Build history of the part. All positions in model axes, mm. Give positions to 0.01 mm unless a question says otherwise; leave off trailing zeros. Order: outer loops, then holes, each group sorted by start corner. A loop starts at its lowest first (then second) coordinate and runs counter-clockwise, first axis right, second up. Notation, with made-up numbers: M -26,52.25 L 5,52.25 A20 cw 5,58.25 Z; hole C 26.25,-8 d8. An arc over 180 degrees is marked long. One line per item, written item: value. Start each with the question number.
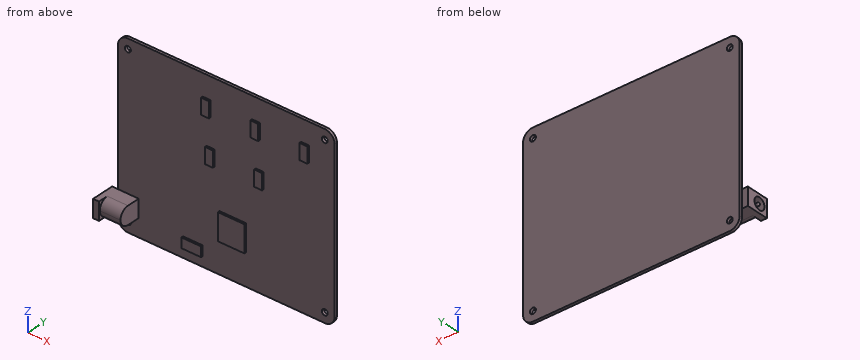
Autodesk Inventor part; units mm, degrees
ref_plane "YZ Plane" through (0, 0, 0) normal (1, 0, 0) x (0, 1, 0)
ref_plane "XZ Plane" through (0, 0, 0) normal (0, 1, 0) x (-1, 0, 0)
ref_plane "XY Plane" through (0, 0, 0) normal (0, 0, 1) x (1, 0, 0)
sketch "草圖1" plane through (0, 0, 0) normal (0, 1, 0) x (-1, 0, 0)
  line L0 (0, 0) -> (110, 0)
  line L1 (110, 0) -> (110, 90)
  line L2 (110, 90) -> (0, 90)
  line L3 (0, 90) -> (0, 0)
  dimension "d0" = 110
  dimension "d1" = 90
extrude "擠出1" add sketch "草圖1" along normal blind 1.4
fillet "圓角1" radius 5 4 edges at (0, 0.7, 90) (0, 0.7, 0) (-110, 0.7, 90) (-110, 0.7, 0)
sketch "草圖2" plane through (0, 0, 0) normal (0, -1, 0) x (1, 0, 0)
  line L0 (-5, 0) -> (-105, 0)
  line L1 (0, 85) -> (0, 5)
  line L2 (-105, 90) -> (-5, 90)
  line L3 (-110, 5) -> (-110, 85)
  point P0 (0, 0)
  point P1 (-105, 85)
  point P2 (-105, 5)
  point P3 (-5, 85)
  point P4 (-5, 5)
  dimension "d5" = 5
  dimension "d6" = 5
  dimension "d7" = 5
  dimension "d8" = 5
hole "孔1" at (-105, 0, 85) at (-105, 0, 5) at (-5, 0, 85) at (-5, 0, 5) direction (0, 1, 0) diameter 3 end through all
sketch "草圖3" plane through (0, 0, 0) normal (0, -1, 0) x (1, 0, 0)
  line L0 (-5, 0) -> (-105, 0)
  line L1 (-110, 5) -> (-110, 85)
  line L2 (-113, 18) -> (-99.5, 18)
  line L3 (-99.5, 18) -> (-99.5, 9)
  line L4 (-99.5, 9) -> (-113, 9)
  line L5 (-113, 9) -> (-113, 18)
  point P0 (0, 0)
  dimension "d16" = 9
  dimension "d17" = 9
  dimension "d18" = 13.5
  dimension "d19" = 3
extrude "擠出2" add sketch "草圖3" along normal blind 11
sketch "草圖5" plane through (0, -11, 0) normal (0, -1, 0) x (1, 0, 0)
  line L0 (-113, 9) -> (-99.5, 9)
  line L1 (-113, 18) -> (-110, 18)
  line L2 (-110, 18) -> (-110, 9)
  line L3 (-110, 9) -> (-113, 9)
  line L4 (-113, 9) -> (-113, 18)
  point P0 (0, 0)
  dimension "d23" = 3
extrude "擠出3" add sketch "草圖5" along normal blind 0.5
fillet "圓角2" radius 4.5 2 edges at (-104.75, -11, 18) (-104.75, -11, 9)
sketch "草圖7" plane through (-113, 0, 9) normal (-1, 0, 0) x (0, 0, 1)
  line L0 (9, -11.5) -> (0, -11.5)
  circle A0 centre (4.5, -7) radius 3
  circle A1 centre (4.5, -7) radius 0.75
  point P0 (-9, 0)
  dimension "d35" = 4.5
  dimension "d36" = 1.5
  dimension "d37" = 6
extrude "擠出4" cut sketch "草圖7" against normal blind 12
fillet "圓角3" radius 0.75 1 edges at (-113, -7, 12.75)
sketch "草圖8" plane through (0, 0, 0) normal (0, -1, 0) x (1, 0, 0)
  line L0 (-5, 0) -> (-105, 0)
  line L1 (0, 85) -> (0, 5)
  line L2 (-105, 90) -> (-5, 90)
  line L3 (-110, 18) -> (-110, 85)
  line L4 (-58.5, 29.5) -> (-45, 29.5)
  line L5 (-45, 29.5) -> (-45, 16)
  line L6 (-45, 16) -> (-58.5, 16)
  line L7 (-58.5, 16) -> (-58.5, 29.5)
  line L8 (-77, 10) -> (-67, 10)
  line L9 (-67, 10) -> (-67, 5)
  line L10 (-67, 5) -> (-77, 5)
  line L11 (-77, 5) -> (-77, 10)
  line L12 (-17, 79) -> (-13, 79)
  line L13 (-13, 79) -> (-13, 71)
  line L14 (-13, 71) -> (-17, 71)
  line L15 (-17, 71) -> (-17, 79)
  line L16 (-38, 79) -> (-42, 79)
  line L17 (-42, 79) -> (-42, 71)
  line L18 (-42, 71) -> (-38, 71)
  line L19 (-38, 71) -> (-38, 79)
  line L20 (-63, 71) -> (-67, 71)
  line L21 (-67, 71) -> (-67, 79)
  line L22 (-67, 79) -> (-63, 79)
  line L23 (-63, 79) -> (-63, 71)
  line L24 (-40, 57) -> (-36, 57)
  line L25 (-36, 57) -> (-36, 49)
  line L26 (-36, 49) -> (-40, 49)
  line L27 (-40, 49) -> (-40, 57)
  line L28 (-65, 57) -> (-61, 57)
  line L29 (-61, 57) -> (-61, 49)
  line L30 (-61, 49) -> (-65, 49)
  line L31 (-65, 49) -> (-65, 57)
  point P0 (0, 0)
  dimension "d41" = 13.5
  dimension "d43" = 13.5
  dimension "d44" = 51.5
  dimension "d45" = 16
  dimension "d46" = 10
  dimension "d47" = 5
  dimension "d48" = 33
  dimension "d49" = 5
  dimension "d50" = 4
  dimension "d51" = 8
  dimension "d52" = 13
  dimension "d53" = 11
  dimension "d54" = 4
  dimension "d55" = 4
  dimension "d56" = 21
  dimension "d57" = 21
  dimension "d58" = 4
  dimension "d59" = 8
  dimension "d60" = 2
  dimension "d61" = 14
  dimension "d62" = 4
  dimension "d63" = 21
extrude "擠出5" add sketch "草圖8" along normal blind 1
properties part number "pcb"
1) Slice it at C-C (x = -19.5). List the corners of the cut face in (y, z).
2) Slice it at B-B (z = 62.5). List the corners of the cut face in (x, y), plus the area to 3 significant figures.
3) Drop flat-ended pins along their axis: P1, Ø0.5, axis at y = -0.5, z = 20.5, coming from the +X side; P2, Ø10, axis at x = -25, z = 72.5, coming from the -Y side; P3, Ø0.8, axis at y = -0.5, z = 74.5, coming from the +X side. Give the stop position or say it passes through.
4) Slice it at A-A (x = -54). List the corners of the cut face in (y, z).
5) Drill centre lines: line 1 (X direction, y = 0.9, z = 85); line 2 (Z direction, x = -5, y = 0.85); line 3 (X direction, y = 0.25, z = 17). Where is each one in solid material? Low to high.
Results list:
1. outline: M 0,0 L 1.4,0 L 1.4,90 L 0,90 Z
2. outline: M -110,0 L 0,0 L 0,1.4 L -110,1.4 Z
2. area: 154 mm²
3. P1: stops at x = -45
3. P2: stops at y = 0
3. P3: stops at x = -13
4. outline: M -1,16 L 0,16 L 0,0 L 1.4,0 L 1.4,90 L 0,90 L 0,29.5 L -1,29.5 Z
5. line 1: x = -110 to -106.5, -103.5 to -6.5, -3.5 to 0
5. line 2: z = 0 to 3.5, 6.5 to 83.5, 86.5 to 90
5. line 3: x = -110 to 0
